from build123d import *

# Parameters (mm, degrees)
EXTRUDE_1_DEPTH      = 27
EXTRUDE_1_DEPTH_BACK = 1


with BuildPart() as part:
    # Эскиз1 → Бобышка-Вытянуть1 (new body, two sides)
    with BuildSketch(Plane.XY) as extrude_1_sk:
        with BuildLine():
            Line((-11.313708499, 4), (-16, 4))
            Line((-16, 4), (-16, -4))
            Line((-16, -4), (-11.313708499, -4))
            ThreePointArc((-11.313708499, -4), (12, 0), (-11.313708499, 4))
        make_face()
        with BuildLine():
            Line((3.31662479, 5), (-3.31662479, 5))
            ThreePointArc((-3.31662479, 5), (-6, 0), (-3.31662479, -5))
            Line((-3.31662479, -5), (3.31662479, -5))
            ThreePointArc((3.31662479, -5), (6, 0), (3.31662479, 5))
        make_face(mode=Mode.SUBTRACT)
    extrude(amount=EXTRUDE_1_DEPTH)
    extrude(extrude_1_sk.sketch, amount=-EXTRUDE_1_DEPTH_BACK)


solid = part.part
Read the model definition and answer for the solid it produces. Units are mm, in the model's axes. A direction names the side the tool comes from. Coordinates: 2 decimals unless noted, no trailing zeros. Order: outer loops, then holes, each group sorted by start corner. A loop starts at its lowest first (then second) coordinate and runs counter-clockwise, first axis right, second up. Notation, with made-up numbers: (-6.5, 36) - (41.5, 36) arc R19 cw to (41.5, 45) - close; hole circle Ø4 at (27.5, 89). An arc over 180 degrees is marked (long way). Use one line per item in the form item = value.
(1) Section D-D, the plane x = -6.5 is taken. Give the vertices of the cut face in (y, z).
Computed values:
outline = (-10.09, -1) - (10.09, -1) - (10.09, 27) - (-10.09, 27) - close
(2) Section C-C, the plane y = 4.5 is taken. Give the vertices of the cut face in (x, z).
Computed values:
outline = (-11.12, -1) - (-3.97, -1) - (-3.97, 27) - (-11.12, 27) - close; (3.97, -1) - (11.12, -1) - (11.12, 27) - (3.97, 27) - close
(3) Section B-B, the plane z = 16.75 is taken. Give the vertices of the cut face in (x, y), then the cut area to 3 significant figures.
Computed values:
outline = (-16, -4) - (-11.31, -4) arc R12 ccw (long way) to (-11.31, 4) - (-16, 4) - close; hole (-3.32, -5) - (3.32, -5) arc R6 ccw to (3.32, 5) - (-3.32, 5) arc R6 ccw to start
area = 382 mm²
(4) Straight lines are drawn through the part: L1, parallel to Y at x = -14.5, z = 15; L2, parallel to X at y = -1.5, z = 3.25; L3, parallel to X at y = 1.75, z = 0.5. For each, find the intervals that lie inside material, in ascending order.
Computed values:
L1 = -4 to 4
L2 = -16 to -5.81, 5.81 to 11.91
L3 = -16 to -5.74, 5.74 to 11.87
(5) Given pin 1 Ø12 at (x, z) = (9, 17) entering from +Y; pin 2 Ø5 at (x, z) = (-9, 6) entering from -Y; pin 3 Ø3.5 at (x, z) = (-14, 8.5) entering from +Y, each flat-ended and moving along its own axis, determine where each tip first touches the part or whether it passes through.
Computed values:
pin_1 = 11.62
pin_2 = -10.09
pin_3 = 4
(6) Which of the six approach directions +Z, -Z, +X, -X, +Y, -Y give full straight-line access (tool end or side, diameter ignored) to faces 1 (the face through (-14, 4, 13)), 2 (the face through (6, 0, 13)), 3 (the face through (-14, -4, 13))?
Computed values:
face_1 = +Z, -Z, -X, +Y
face_2 = +Z, -Z
face_3 = +Z, -Z, -X, -Y
(7) For a pull along Y with two mould halves and no side action, classify faces 4 (the face through (0, 5, 13)), 5 (the face through (-2.2, -5.2, 27)), 6 (the face through (12, 0, 13)) as pulls with the +Y half, pulls with the -Y half, needs draft (parallel to the pull), parting line crosses it, or undercut.
Computed values:
face_4 = undercut
face_5 = needs draft
face_6 = parting line crosses it
(8) Section A-A, the plane x = 0 is taken. Give the vertices of the cut face in (y, z), then the cut area to 3 significant figures.
Computed values:
outline = (-12, -1) - (-5, -1) - (-5, 27) - (-12, 27) - close; (5, -1) - (12, -1) - (12, 27) - (5, 27) - close
area = 392 mm²
